Source: CAD feature listing. Evaluate the final solid. Frame: model axes, mm. A direction names the side the tool comes from. Coordinates: 2 decimals unless noted, no trailing zeros. Order: outer loops, then holes, each group sorted by start corner. A loop starts at its lowest first (then second) coordinate and runs counter-clockwise, first axis right, second up.
Autodesk Inventor part; units mm, degrees
ref_plane "YZ Plane" through (0, 0, 0) normal (1, 0, 0) x (0, 1, 0)
ref_plane "XZ Plane" through (0, 0, 0) normal (0, 1, 0) x (-1, 0, 0)
ref_plane "XY Plane" through (0, 0, 0) normal (0, 0, 1) x (1, 0, 0)
sketch "Sketch1" plane through (0, 0, 0) normal (0, 0, 1) x (1, 0, 0)
  line L0 (-50.8, 66.75) -> (50.8, 66.75)
  line L1 (50.8, 66.75) -> (50.8, -66.6)
  line L2 (50.8, -66.6) -> (-50.8, -66.6)
  line L3 (-50.8, -66.6) -> (-50.8, 66.75)
  point P0 (0, 0)
  dimension "d1" = 101.6
  dimension "d2" = 133.35
  dimension "d3" = 66.75
  dimension "d4" = 50.8
extrude "Extrusion1" add sketch "Sketch1" along normal blind 100.075
sketch "Sketch2" plane through (0, 0, 100.075) normal (0, 0, 1) x (1, 0, 0)
  circle A0 centre (0, 0) radius 13.625
  dimension "d7" = 27.25
extrude "Extrusion2" add sketch "Sketch2" along normal blind 38.1
sketch "Sketch3" plane through (0, 0, 0) normal (0, 0, -1) x (-1, 0, 0)
  circle A0 centre (0, 0) radius 31.75
  dimension "d10" = 63.5
extrude "Extrusion3" add sketch "Sketch3" along normal blind 82.55
sketch "Sketch4" plane through (50.8, -66.6, 0) normal (1, 0, 0) x (0, 0, -1)
  line L0 (0, 133.35) -> (-100.075, 133.35)
  line L1 (-81.787, 133.35) -> (-18.288, 133.35)
  line L2 (-18.288, 133.35) -> (-18.288, 69.851)
  line L3 (-18.288, 69.851) -> (-81.787, 69.851)
  line L4 (-81.787, 69.851) -> (-81.787, 133.35)
  line L5 (0, 133.35) -> (0, 0)
  line L6 (-100.075, 0) -> (-100.075, 133.35)
  line L7 (0, 0) -> (-100.075, 0)
  line L8 (-81.787, 0) -> (-18.288, 0)
  line L9 (-18.288, 0) -> (-18.288, 63.499)
  line L10 (-18.288, 63.499) -> (-81.787, 63.499)
  line L11 (-81.787, 63.499) -> (-81.787, 0)
  point P0 (0, 66.6)
  dimension "d13" = 18.288
  dimension "d14" = 18.288
  dimension "d15" = 63.499
  dimension "d16" = 63.499
  dimension "d17" = 63.499
extrude "Extrusion4" add sketch "Sketch4" along normal blind 90.424 contours L2 L3 L4 L0 | L7 L11 L10 L9
sketch "Sketch5" plane through (-50.8, -66.6, 0) normal (-1, 0, 0) x (0, 0, 1)
  line L0 (18.288, 69.851) -> (18.288, 133.35)
  line L1 (18.288, 69.851) -> (81.787, 69.851)
  line L2 (18.288, 133.35) -> (81.787, 133.35)
  line L3 (81.787, 133.35) -> (81.787, 69.851)
  line L4 (81.787, 69.851) -> (18.288, 69.851)
  line L5 (18.288, 69.851) -> (18.288, 133.35)
  line L6 (18.288, 0) -> (18.288, 63.499)
  line L7 (81.787, 0) -> (81.787, 63.499)
  line L8 (18.288, 63.499) -> (81.787, 63.499)
  line L9 (81.787, 63.499) -> (81.787, 0)
  line L10 (81.787, 0) -> (18.288, 0)
  line L11 (18.288, 0) -> (18.288, 63.499)
  point P0 (0, 66.6)
extrude "Extrusion5" add sketch "Sketch5" along normal blind 90.424
equation "\"d16\" = d15"
equation "\"d17\" = d15"
properties part number "Semi Rotary Hydraulic Motor"
1. Material intervals for line 1 along Y through (x, z) = (62.5, 70); line 2 along Z through (x, y) = (-39.5, 50) (3 decimals); line 3 along Z through (x, y) = (88, 14.5), sorted ascending.
2. Section query C-C, the plane z = 61.5. Output: boundary loops of the cut face in (x, y), plus the area to 3 significant figures.
3. Section query A-A, the plane x = 122. Output: boundary loops of the cut face in (y, z), plus the area to 3 significant figures.
4. Draft query along Y for faces 4 (the flat face through (141.224, -34, 50)), 5 (the cylindrical face through (-10.812, 8.291, 118.858)), 6 (the flat face through (50.8, 1, 49)). Return one class per face: +Y half, -Y half, draft (parallel to the pull), parting line (faces both ways), or undercut.
5. Section query D-D, the plane y = -19. Output: boundary loops of the cut face in (x, z) (3 decimals).
6. Section query B-B, the plane x = 0. Output: boundary loops of the cut face in (y, z) (3 decimals).
7. Access query for faces 1 (the flat face through (95, -35, 18.288)), 2 (the flat face through (11, 31, 0)), 3 (the flat face through (95, -3.101, 50)). Directions: +Z, -Z, +X, -X, +Y, -Y. A direction counts if a zero-diameter tool reaches every point of the face in a straight line with its end or side. Return the directions, or none.
8. Contact query for flat-ended pins moving along their axis: P1, Ø12, axis at y = 0, z = 102, coming from the -X side; P2, Ø1.5, axis at x = 102, y = -46, coming from the +Z side; P3, Ø8, axis at x = 95.5, z = 89, coming from the +Y side; P4, Ø1, axis at x = 39, y = -17, coming from the -Z side. Output: stop coordinate, or through.
Answer key:
1. line 1: y = -66.6 to -3.1, 3.25 to 66.75
1. line 2: z = 0 to 100.075
1. line 3: z = 18.29 to 81.79
2. outline: (-141.22, -66.6) - (141.22, -66.6) - (141.22, -3.1) - (50.8, -3.1) - (50.8, 3.25) - (141.22, 3.25) - (141.22, 66.75) - (-141.22, 66.75) - (-141.22, 3.25) - (-50.8, 3.25) - (-50.8, -3.1) - (-141.22, -3.1) - close
2. area: 36,500 mm2
3. outline: (-66.6, 18.29) - (-3.1, 18.29) - (-3.1, 81.79) - (-66.6, 81.79) - close; (3.25, 18.29) - (66.75, 18.29) - (66.75, 81.79) - (3.25, 81.79) - close
3. area: 8,060 mm2
4. face 4: draft
4. face 5: parting line
4. face 6: undercut
5. outline: (-141.224, 18.288) - (-50.8, 18.288) - (-50.8, 0) - (-25.437, 0) - (-25.437, -82.55) - (25.437, -82.55) - (25.437, 0) - (50.8, 0) - (50.8, 18.288) - (141.224, 18.288) - (141.224, 81.787) - (50.8, 81.787) - (50.8, 100.075) - (-50.8, 100.075) - (-50.8, 81.787) - (-141.224, 81.787) - close
6. outline: (-66.6, 0) - (-31.75, 0) - (-31.75, -82.55) - (31.75, -82.55) - (31.75, 0) - (66.75, 0) - (66.75, 100.075) - (13.625, 100.075) - (13.625, 138.175) - (-13.625, 138.175) - (-13.625, 100.075) - (-66.6, 100.075) - close
7. face 1: -Z, +X, +Y, -Y
7. face 2: -Z
7. face 3: +Z, -Z, +X
8. P1: stops at x = -50.8
8. P2: stops at z = 81.79
8. P3: passes through
8. P4: stops at z = 0
